Could you check a few things on this model? Use its own coordinates, in mm. A direction names the side the tool comes from. Round coordinates to 2 decimals unless told otherwise and drop trailing zeros. Order: outer loops, then holes, each group sorted by start corner. A loop starts at its lowest first (then second) coordinate and runs counter-clockwise, first axis right, second up. Notation, with made-up numbers: (59, 49) -> (107, 49) arc R12 cw to (107, 60) -> close; hole circle Ø2 at (40.5, 70.5). An arc over 180 degrees is marked (long way). Put each result on its own line as item: value. Start each with the question number.
Autodesk Inventor part; units mm, degrees
ref_plane "YZ Plane" through (0, 0, 0) normal (1, 0, 0) x (0, 1, 0)
ref_plane "XZ Plane" through (0, 0, 0) normal (0, 1, 0) x (-1, 0, 0)
ref_plane "XY Plane" through (0, 0, 0) normal (0, 0, 1) x (1, 0, 0)
ref_plane "Work Plane1" through (0, 0, 0) normal (0, 0, 1) x (1, 0, 0)
sketch "Sketch1" plane through (0, 0, 0) normal (0, 0, 1) x (1, 0, 0)
  line L0 (5.0907, -20) -> (5.0907, 0)
  line L1 (25.0907, -20) -> (5.0907, -20)
  line L2 (25.0907, 0) -> (25.0907, -20)
  line L3 (5.0907, 0) -> (25.0907, 0)
  line L4 (5.0907, 71.5801) -> (25.0907, 71.5801)
  line L5 (5.0907, 91.5801) -> (25.0907, 91.5801)
  line L6 (5.0907, 91.5801) -> (5.0907, 71.5801)
  line L7 (24.826, 92.0223) -> (24.826, 72.0223)
  line L8 (2.3907, 2.7) -> (27.7907, 2.7)
  line L9 (27.7907, 2.7) -> (27.7907, -22.7)
  line L10 (27.7907, -22.7) -> (2.3907, -22.7)
  line L11 (2.3907, -22.7) -> (2.3907, 2.7)
  line L12 (2.3907, 2.7) -> (27.7907, -22.7) construction
  line L13 (27.7907, 2.7) -> (2.3907, -22.7) construction
  line L14 (2.3907, 94.7223) -> (27.7907, 94.7223)
  line L15 (27.7907, 94.7223) -> (27.7907, 69.3223)
  line L16 (27.7907, 69.3223) -> (2.3907, 69.3223)
  line L17 (2.3907, 69.3223) -> (2.3907, 94.7223)
  line L18 (2.3907, 94.7223) -> (27.7907, 69.3223) construction
  line L19 (27.7907, 94.7223) -> (2.3907, 69.3223) construction
  line L20 (25.0907, 72.0223) -> (5.0907, 72.0223)
  line L21 (5.0907, 72.0223) -> (5.0907, 92.0223)
  line L22 (5.0907, 92.0223) -> (25.0907, 92.0223)
  line L23 (25.0907, 92.0223) -> (25.0907, 72.0223)
  line L24 (25.0907, 72.0223) -> (5.0907, 92.0223) construction
  line L25 (5.0907, 72.0223) -> (25.0907, 92.0223) construction
  point P0 (0, 0)
  point P1 (15.0907, -10)
  point P2 (15.0907, 82.0223)
  dimension "d0" = 25.4
  dimension "d1" = 25.4
  dimension "d2" = 25.4
  dimension "d3" = 25.4
  dimension "d4" = 20
  dimension "d5" = 20
extrude "Extrusion1" add sketch "Sketch1" along normal blind 50
sketch "Sketch2" plane through (27.7907, 69.3223, 0) normal (1, 0, 0) x (0, 0, -1)
  line L0 (0, 25.4) -> (0, 0)
  line L1 (0, 25.4) -> (-50, 25.4)
  line L2 (-50, 0) -> (-50, 25.4)
  line L3 (0, 0) -> (-50, 0)
  line L4 (0, -66.6223) -> (0, -92.0223)
  line L5 (0, -66.6223) -> (-50, -66.6223)
  line L6 (-50, -92.0223) -> (-50, -66.6223)
  line L7 (0, -92.0223) -> (-50, -92.0223)
  line L8 (0, 25.4) -> (-50, 25.4)
  line L9 (0, 25.4) -> (-50, 25.4)
  line L10 (-50, 25.4) -> (-50, -92.0223)
  line L11 (-50, -92.0223) -> (0, -92.0223)
  line L12 (0, -92.0223) -> (0, 25.4)
  point P0 (0, -69.3223)
extrude "Extrusion2" add sketch "Sketch2" against normal blind 5.08 contours L12 L5 L10 L3
sketch "Sketch3" plane through (22.7107, 69.3223, 0) normal (-1, 0, 0) x (0, 0, 1)
  line L0 (0, 25.4) -> (0, -92.0223)
  line L1 (0, 25.4) -> (50, 25.4)
  line L2 (50, -92.0223) -> (50, 25.4)
  line L3 (0, -92.0223) -> (50, -92.0223)
  circle A0 centre (25, -33.3111) radius 12.5
  line L4 (25, -33.3111) -> (9.5, -33.3111)
  line L5 (9.5, -33.3111) -> (9.5, -48.8111)
  circle A1 centre (9.5, -48.8111) radius 2
  circle A2 centre (9.5, -17.8111) radius 2
  circle A3 centre (40.5, -48.8111) radius 2
  circle A4 centre (40.5, -17.8111) radius 2
  point P0 (0, -69.3223)
  dimension "d10" = 25
  dimension "d11" = 15.5
  dimension "d12" = 15.5
  dimension "d13" = 4
  dimension "d16" = 31
  dimension "d19" = 31
extrude "Extrusion3" cut sketch "Sketch3" against normal blind 5.08 contours A0 | A1 | A2 | A3 | A4
properties part number "ExtruderMount"
1. I need wall thicknesses on L1, parallel to Y at x = 24.45, z = 25; L2, parallel to Y at x = 13.75, z = 33; L3, parallel to Y at x = 24.7, z = 9.5. Which ranges of each line are inside material? Lowest first, please.
2. Which directions (+Z, -Z, +X, -X, +Y, -Y) give clear straight access to the entire face, cutting with the end or side of a thin tool? Please do faces 1 (the face through (25.22, 18.56, 40.07)), 2 (the face through (13, 69.322, 25)), 3 (the face through (15, 72.022, 25)).
3. For pin 1 Ø3 at (y, z) = (25.5, 24) entering from -X (3 decimals); pin 2 Ø6.5 at (y, z) = (20.51, 9.5) entering from +X, each with a flat end and sliding along its axis, tell me the tip position at first contact or that it passes through.
4. If we section it at C-C, the plane x = 7.75: Please give me the cut outline in (y, z).
5. If we section it at D-D, the plane z = 40.5: Please give me the cut outline in (x, y).
6. If we section it at A-A, the plane z = 25: Please give me the cut outline in (x, y), then the cut area to 3 significant figures.
7. If we section it at B-B, the plane y = 75: Please give me the cut outline in (x, z), then the cut area to 3 significant figures.
8. Thinking about a two-plate mould opening in X: for faces 4 (the face through (2.391, -10, 25)), 5 (the face through (27.791, 50, 25)), 6 (the face through (25.22, 18.56, 9.07)), 7 (the face through (25.091, 82, 25)), which applies, +X half, -X half, draft (parallel to the pull), parting line (faces both ways), or undercut?
Results below:
1. L1: -22.7 to -20, 0 to 23.51, 48.51 to 72.02, 92.02 to 94.72
1. L2: -22.7 to -20, 0 to 2.7, 69.32 to 72.02, 92.02 to 94.72
1. L3: -22.7 to -20, 0 to 18.51, 22.51 to 49.51, 53.51 to 72.02, 92.02 to 94.72
2. face 1: +X, -X
2. face 2: +Z, -Z, -X
2. face 3: +Z, -Z
3. pin 1: through
3. pin 2: x = 27.79
4. outline: (-22.7, 0) -> (-20, 0) -> (-20, 50) -> (-22.7, 50) -> close; (0, 0) -> (2.7, 0) -> (2.7, 50) -> (0, 50) -> close; (69.32, 0) -> (72.02, 0) -> (72.02, 50) -> (69.32, 50) -> close; (92.02, 0) -> (94.72, 0) -> (94.72, 50) -> (92.02, 50) -> close
5. outline: (2.39, -22.7) -> (27.79, -22.7) -> (27.79, 18.51) -> (22.71, 18.51) -> (22.71, 2.7) -> (2.39, 2.7) -> close; (2.39, 69.32) -> (22.71, 69.32) -> (22.71, 53.51) -> (27.79, 53.51) -> (27.79, 94.72) -> (2.39, 94.72) -> close; (22.71, 22.51) -> (27.79, 22.51) -> (27.79, 49.51) -> (22.71, 49.51) -> close; hole (5.09, -20) -> (25.09, -20) -> (25.09, 0) -> (5.09, 0) -> close; hole (5.09, 72.02) -> (25.09, 72.02) -> (25.09, 92.02) -> (5.09, 92.02) -> close
6. outline: (2.39, -22.7) -> (27.79, -22.7) -> (27.79, 23.51) -> (22.71, 23.51) -> (22.71, 2.7) -> (2.39, 2.7) -> close; (2.39, 69.32) -> (22.71, 69.32) -> (22.71, 48.51) -> (27.79, 48.51) -> (27.79, 94.72) -> (2.39, 94.72) -> close; hole (5.09, -20) -> (25.09, -20) -> (25.09, 0) -> (5.09, 0) -> close; hole (5.09, 72.02) -> (25.09, 72.02) -> (25.09, 92.02) -> (5.09, 92.02) -> close
6. area: 702 mm2
7. outline: (2.39, 0) -> (5.09, 0) -> (5.09, 50) -> (2.39, 50) -> close; (25.09, 0) -> (27.79, 0) -> (27.79, 50) -> (25.09, 50) -> close
7. area: 270 mm2
8. face 4: -X half
8. face 5: +X half
8. face 6: draft
8. face 7: undercut
